For this review, take the finished solid that the model builds, in its own axes (mm). A direction names the side the tool comes from. Coordinates: 2 decimals unless noted, no trailing zeros. Use one line per item in the form item = value.
```python
from build123d import *

# Parameters (mm, degrees)
FILLET_1_R = 0.8


with BuildPart() as part:
    # Эскиз1 → Повернуть1 (revolve)
    with BuildSketch(Plane.XY, mode=Mode.PRIVATE) as revolve_1_sk:
        Polygon((3.5, 10), (-3.5, 10), (-3.5, 11.5), (-3, 11.5), (-3, 14.5), (-3.5, 14.5), (-3.5, 16), (3.5, 16), (3.5, 14.5), (3, 14.5), (3, 11.5), (3.5, 11.5), align=None)
    revolve(revolve_1_sk.sketch.rotate(Axis((0, 0, 0), (-1, 0, 0)), 90), axis=Axis((0, 0, 0), (-1, 0, 0)))

    # Скругление1
    fillet_1_edges = [part.edges().sort_by_distance(p)[0] for p in [
        (-3.5, 0, 16),
        (3.5, 0, 16),
        (3.5, 0, 10),
        (-3.5, 0, 10),
    ]]
    fillet(fillet_1_edges, radius=FILLET_1_R)


solid = part.part
```
1. Draft analysis for pull direction Z (two halves, no side actions). For faces 1 (the face through (-3.2, -11.4, 1.5)), 2 (the face through (0.04, 15.62, 3.47)), 3 (the face through (-3.5, 15, 0)), state which applies: +Z half, -Z half, draft (parallel to the pull), parting line (faces both ways), or undercut.
Computed values:
face_1 = undercut
face_2 = parting line
face_3 = draft
2. Tool access review of faces 4 (the face through (-3, -8, -9)), 5 (the face through (0, 0, 10)), 6 (the face through (3.3, -11.4, 1.5)): name each direction out of +Z, -Z, +X, -X, +Y, -Y from which nothing blocks a thin tool from reaching the whole face with its end or side.
Computed values:
face_4 = -X
face_5 = +X, -X
face_6 = +X
3. For pin 1 Ø8.5 at (y, z) = (-5.5, 0) entering from +X; pin 2 Ø1 at (x, z) = (-1.5, -4) entering from +Y; pin 3 Ø1 at (y, z) = (-10, -6.5) entering from -X; pin 4 Ø1.5 at (x, y) = (3, -6) entering from +Z, all flat-tipped, find the tip position at first contact; note any pin that passes through.
Computed values:
pin_1 = through
pin_2 = 15.61
pin_3 = -3.5
pin_4 = 15.1
4. Wall thickness on line 1 along Y through (x, z) = (3.25, -9); line 2 along Y through (x, z) = (-0.85, 0); line 3 along Y through (x, z) = (-2.25, 3.5): over which ranges is each line inside the solid? List them lowest first. Write a range as from..to.
Computed values:
line_1 = -12.96..-11.37, -7.16..-4.84, 4.84..7.16, 11.37..12.96
line_2 = -16..-10, 10..16
line_3 = -15.61..-9.37, 9.37..15.61
